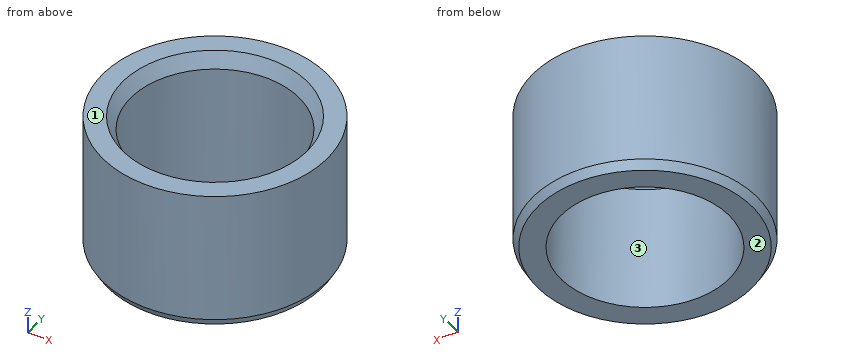
from build123d import *

# Parameters (mm, degrees)
SKETCH1_R           = 4
SKETCH1_R_2         = 3
BOSS_EXTRUDE1_DEPTH = 5
CHAMFER1_SIZE       = 0.3
CHAMFER1_SIZE2      = 0.173205081
CHAMFER2_SIZE       = 0.5
CHAMFER2_SIZE2      = 0.288675135


with BuildPart() as part:
    # Sketch1 → Boss-Extrude1 (new body)
    with BuildSketch(Plane.XY):
        Circle(SKETCH1_R)
        Circle(SKETCH1_R_2, mode=Mode.SUBTRACT)
    extrude(amount=BOSS_EXTRUDE1_DEPTH)

    # Chamfer1
    chamfer1_edges = [part.edges().sort_by_distance(p)[0] for p in [
        (-4, 0, 0),
    ]]
    chamfer1_side = [part.faces().sort_by_distance(p)[0] for p in [
        (-4, 0, 2.5),
    ]]
    chamfer(chamfer1_edges, length=CHAMFER1_SIZE, length2=CHAMFER1_SIZE2, reference=chamfer1_side[0])

    # Chamfer2
    chamfer2_edges = [part.edges().sort_by_distance(p)[0] for p in [
        (-3, 0, 5),
    ]]
    chamfer2_side = [part.faces().sort_by_distance(p)[0] for p in [
        (-3, 0, 2.5),
    ]]
    chamfer(chamfer2_edges, length=CHAMFER2_SIZE, length2=CHAMFER2_SIZE2, reference=chamfer2_side[0])


solid = part.part
Input: part model. Units: mm. Frame: model coordinates. Face numbers are marked on the shaded views. Give positions to 0.01 mm unless a question says otherwise; leave off trailing zeros. Loops run counter-clockwise (first coordinate to the right, second up) from the corner with the lowest first, then second, coordinate; pieces in that order, holes last. Notation, with made-up numbers: (16, 56) - (64, 56) arc R17 cw to (64, 66) - close; hole circle Ø10 at (69.25, -2.75). An arc over 180 degrees is marked (long way). Use CSV: the item, a comma, the result in double quotes. Start each with the question number.
Item 1: Line query: line 1 (Y direction, x = 0, z = 2.6); line 2 (Y direction, x = 1, z = 3.8); line 3 (X direction, y = 2.75, z = 0.75). Output: solid intervals per line, ascending.
Item 2: Section A-A on x = 0. Return loops of the section in (y, z).
Item 3: Section C-C on z = 1.8. Return loops of the section in (x, y), then the cut area to 3 significant figures.
Item 4: Contact query for flat-ended pins moving along their axis: P1, Ø3, axis at x = -1, y = 2.5, coming from the +Z side; P2, Ø3, axis at y = 2.5, z = 1.5, coming from the -X side; P3, Ø2, axis at x = -1.5, z = 3, coming from the -Y side. Output: stop coordinate, or through.
Item 5: Mould query, pull axis Z, two halves, no side actions, for the marked faces 1, 2 and 3. Classes: pulls with the +Z half, pulls with the -Z half, needs draft (parallel to the pull), parting line crosses it, or undercut.
Ans:
1,line 1,"y = -4 to -3, 3 to 4"
1,line 2,"y = -3.87 to -2.83, 2.83 to 3.87"
1,line 3,"x = -2.9 to -1.2, 1.2 to 2.9"
2,outline,"(-4, 0.3) - (-3.83, 0) - (-3, 0) - (-3, 4.5) - (-3.29, 5) - (-4, 5) - close; (3, 0) - (3.83, 0) - (4, 0.3) - (4, 5) - (3.29, 5) - (3, 4.5) - close"
3,outline,"circle Ø8 at (0, 0); hole circle Ø6 at (0, 0)"
3,area,"22.0 mm2"
4,P1,"stops at z = 5"
4,P2,"stops at x = -3.87"
4,P3,"stops at y = -3.97"
5,face 1,"pulls with the +Z half"
5,face 2,"pulls with the -Z half"
5,face 3,"needs draft"
